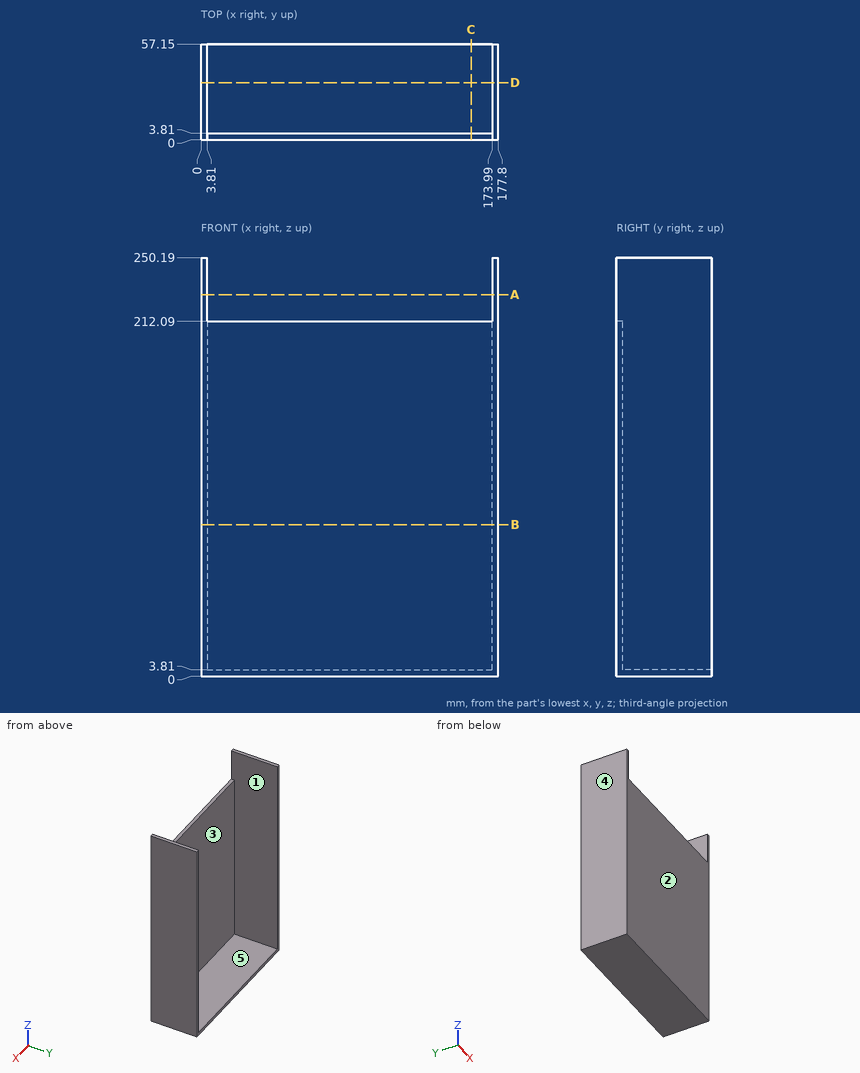
For this review, use the dimensioned drawing (mm, ordinates from the lowest corner) and the shaded views. A direction names the side the tool comes from. Coordinates: 2 decimals unless noted, no trailing zeros. Write each loop counter-clockwise with the first axis right and the second up, starting at its lowest first coordinate (ties: lowest second). Pieces come first, ordered by that corner, then holes. Notation, with made-up numbers: (46.25, 72) - (85.25, 72) arc R35 ccw to (85.25, 105) - close; hole circle Ø9 at (3.25, 54). An arc over 180 degrees is marked (long way). Answer in a Markdown table with one row per item. Add a question column.
Q1. Consider section C-C on x = 161.5. Give the boundary of the cut face in (y, z).
Q2. To check wall thickness, follow line 1 along X through (y, z) = (22.5, 177); line 2 along Z through (x, y) = (29.5, 38). State the ranges of each line that lie inside material, in increasing order. Write a range as from..to.
Q3. Consider section B-B on z = 90.5. Give the boundary of the cut face in (x, y).
Q4. Clearance check with flat-ended pins moving along their axes: pin 1 (5 mm diameter, centred on x = 31, z = 140.5, fed in from +Y); pin 2 (1.9 mm diameter, centred on x = 112.5, y = 2.5, fed in from +Z); pin 3 (1 mm diameter, centred on x = 67.5, y = 8, fed in from +Z); pin 4 (1.5 mm diameter, centred on y = 7.5, z = 57.5, fed in from -X). State where each tip first meets the part, or that it passes through.
Q5. Consider section A-A on z = 228. Give the boundary of the cut face in (x, y), then the cut area to 3 significant figures.
Q6. Consider section D-D on y = 34. Give the boundary of the cut face in (x, z).
Q7. Draft analysis for pull direction Y (two halves, no side actions). For the marked faces 1, 2 and 3, state which applies: +Y half, -Y half, draft (parallel to the pull), parting line (faces both ways), or undercut.
Q8. For the marked faces 4 and 5, list the 3-axis set-ups (+Z, -Z, +X, -X, +Y, -Y) from which the entire face can be reached by the end or side of a thin tool; tool diameter is ignored.
Answers below:
| question | item | result |
|---|---|---|
| 1 | outline | (0, 0) - (57.15, 0) - (57.15, 3.81) - (3.81, 3.81) - (3.81, 212.09) - (0, 212.09) - close |
| 2 | line 1 | 0..3.81, 173.99..177.8 |
| 2 | line 2 | 0..3.81 |
| 3 | outline | (0, 0) - (177.8, 0) - (177.8, 57.15) - (173.99, 57.15) - (173.99, 3.81) - (3.81, 3.81) - (3.81, 57.15) - (0, 57.15) - close |
| 4 | pin 1 | y = 3.81 |
| 4 | pin 2 | z = 212.09 |
| 4 | pin 3 | z = 3.81 |
| 4 | pin 4 | x = 0 |
| 5 | outline | (0, 0) - (3.81, 0) - (3.81, 57.15) - (0, 57.15) - close; (173.99, 0) - (177.8, 0) - (177.8, 57.15) - (173.99, 57.15) - close |
| 5 | area | 435 mm² |
| 6 | outline | (0, 0) - (177.8, 0) - (177.8, 250.19) - (173.99, 250.19) - (173.99, 3.81) - (3.81, 3.81) - (3.81, 250.19) - (0, 250.19) - close |
| 7 | face 1 | draft |
| 7 | face 2 | -Y half |
| 7 | face 3 | +Y half |
| 8 | face 4 | +Z, -Z, -X, +Y, -Y |
| 8 | face 5 | +Z, +Y |
